Source: CAD feature listing. Evaluate the final solid. Frame: model axes, mm. Face numbers are marked on the shaded views. A direction names the side the tool comes from. Coordinates: 2 decimals unless noted, no trailing zeros. Order: outer loops, then holes, each group sorted by start corner. A loop starts at its lowest first (then second) coordinate and runs counter-clockwise, first axis right, second up. Notation, with made-up numbers: (34.25, -17) - (57.25, -17) arc R21 cw to (57.25, 5) - close; hole circle Ø7 at (-8, 13). An arc over 180 degrees is marked (long way). One line per question, with ' | ' between items.
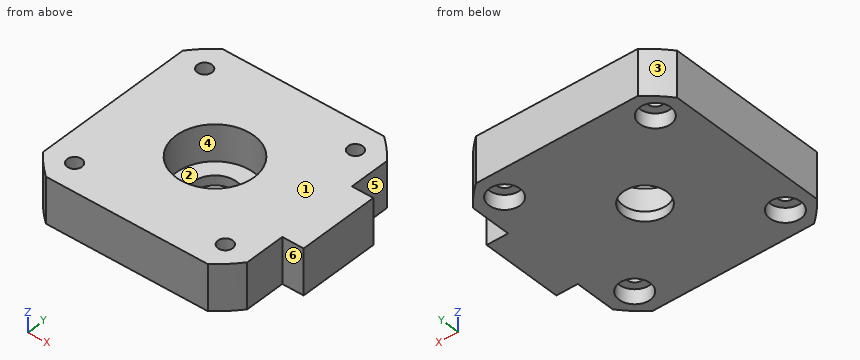
from build123d import *

# Parameters (mm, degrees)
SKETCH_R        = 4.5
SKETCH_R_2      = 1.5
PAD_DEPTH       = 9.4
SKETCH002_R     = 3.2
POCKET_DEPTH    = 3
SKETCH003_R     = 8
POCKET001_DEPTH = 8


with BuildPart() as part:
    # Sketch → Pad (new body)
    with BuildSketch(Plane.XY):
        with BuildLine():
            ThreePointArc((-16.650526, 21), (-18.950462, 18.950462), (-21, 16.650526))
            Line((-21, 16.650526), (-21, -16.650526))
            ThreePointArc((-21, -16.650526), (-18.950462, -18.950462), (-16.650526, -21))
            Line((-16.650526, -21), (16.650526, -21))
            ThreePointArc((16.650526, -21), (18.950462, -18.950462), (21, -16.650526))
            Line((21, -8.3), (21, -16.650526))
            Line((25.4, -8.3), (21, -8.3))
            Line((25.4, 8.3), (25.4, -8.3))
            Line((21, 8.3), (25.4, 8.3))
            Line((21, 16.650526), (21, 8.3))
            ThreePointArc((21, 16.650526), (18.950462, 18.950462), (16.650526, 21))
            Line((-16.650526, 21), (16.650526, 21))
        make_face()
        Circle(SKETCH_R, mode=Mode.SUBTRACT)
        with Locations((-15.5, 15.5)):
            Circle(SKETCH_R_2, mode=Mode.SUBTRACT)
        with Locations((15.5, 15.5)):
            Circle(SKETCH_R_2, mode=Mode.SUBTRACT)
        with Locations((15.5, -15.5)):
            Circle(SKETCH_R_2, mode=Mode.SUBTRACT)
        with Locations((-15.5, -15.5)):
            Circle(SKETCH_R_2, mode=Mode.SUBTRACT)
    extrude(amount=PAD_DEPTH)

    # Sketch002 → Pocket (cut)
    with BuildSketch(Plane.XY):
        with Locations((-15.5, 15.5)):
            Circle(SKETCH002_R)
        with Locations((15.5, 15.5)):
            Circle(SKETCH002_R)
        with Locations((15.5, -15.5)):
            Circle(SKETCH002_R)
        with Locations((-15.5, -15.5)):
            Circle(SKETCH002_R)
    extrude(amount=POCKET_DEPTH, mode=Mode.SUBTRACT)

    # Sketch003 → Pocket001 (cut)
    with BuildSketch(Plane.XY.offset(10)):
        Circle(SKETCH003_R)
    extrude(amount=-POCKET001_DEPTH, mode=Mode.SUBTRACT)


solid = part.part
(1) Cut plane D-D (x = 0). Return the cut outline in (y, z), and give its area (3 significant figures).
Taken from the geometry:
outline: (-21, 0) - (-4.5, 0) - (-4.5, 2) - (-8, 2) - (-8, 9.4) - (-21, 9.4) - close; (4.5, 0) - (21, 0) - (21, 9.4) - (8, 9.4) - (8, 2) - (4.5, 2) - close | area: 258 mm²
(2) Pin query (flat end, axial travel): P1, Ø1.9, axis at x = 16, y = -14, coming from the -Z side; P2, Ø2.5, axis at x = -15.5, y = -15.5, coming from the +Z side; P3, Ø2, axis at x = 23.5, z = 3.5, coming from the -Y side; P4, Ø4, axis at x = 19.5, z = 2.5, coming from the +Y side. Return the tip coordinate at first contact, or that it passes through.
Taken from the geometry:
P1: stops at z = 3 | P2: passes through | P3: stops at y = -8.3 | P4: stops at y = 20.3
(3) Cut plane A-A (y = 15.5). Return the cut outline in (x, z), and give its area (3 significant figures).
Taken from the geometry:
outline: (-21, 0) - (-18.7, 0) - (-18.7, 3) - (-17, 3) - (-17, 9.4) - (-21, 9.4) - close; (-14, 3) - (-12.3, 3) - (-12.3, 0) - (12.3, 0) - (12.3, 3) - (14, 3) - (14, 9.4) - (-14, 9.4) - close; (17, 3) - (18.7, 3) - (18.7, 0) - (21, 0) - (21, 9.4) - (17, 9.4) - close | area: 318 mm²
(4) Cut plane C-C (z = 5.25). Return the cut outline in (x, y).
Taken from the geometry:
outline: (-21, -16.65) arc R26.8 ccw to (-16.65, -21) - (16.65, -21) arc R26.8 ccw to (21, -16.65) - (21, -8.3) - (25.4, -8.3) - (25.4, 8.3) - (21, 8.3) - (21, 16.65) arc R26.8 ccw to (16.65, 21) - (-16.65, 21) arc R26.8 ccw to (-21, 16.65) - close; hole circle Ø3 at (-15.5, -15.5); hole circle Ø3 at (-15.5, 15.5); hole circle Ø16 at (0, 0); hole circle Ø3 at (15.5, -15.5); hole circle Ø3 at (15.5, 15.5)
(5) Pull-direction query (Y, two-part tool) for the marked faces 1, 2 and 3; classes: pulls with the +Y half, pulls with the -Y half, needs draft (parallel to the pull), parting line crosses it, or undercut.
Taken from the geometry:
face 1: needs draft | face 2: undercut | face 3: pulls with the +Y half
(6) Set-up query: the marked faces 4, 5 and 6. Return all of +Z, -Z, +X, -X, +Y, -Y with unobstructed straight access to the full face (end or side cutting, diameter ignored); none if empty.
Taken from the geometry:
face 4: +Z | face 5: +Z, -Z, +X, +Y | face 6: +Z, -Z, +X, -Y
(7) Material intervals for L1, parallel to Y at x = 15.5, z = 8; L2, parallel to Y at x = 15.5, z = 2.35, sorted ascending. Write a range as from..to.
Taken from the geometry:
L1: y = -21..-17, -14..14, 17..21 | L2: y = -21..-18.7, -12.3..12.3, 18.7..21
